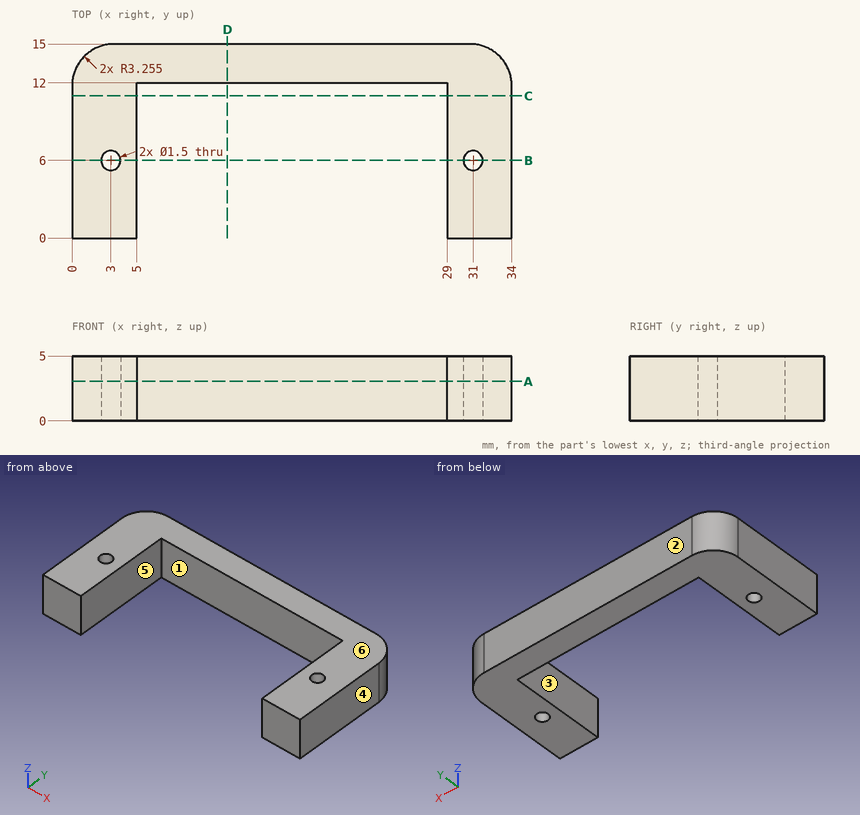
The drawing under review shows one solid part. Ordinate dimensions are in mm from its lowest x, y, z. A direction names the side the tool comes from. Give positions to 0.01 mm unless a question says otherwise; leave off trailing zeros. Order: outer loops, then holes, each group sorted by start corner. A loop starts at its lowest first (then second) coordinate and runs counter-clockwise, first axis right, second up. Notation, with made-up numbers: (66.25, -31) - (102.25, -31) arc R21 cw to (102.25, -25) - close; hole circle Ø7 at (-6.75, -29). An arc over 180 degrees is marked (long way). Answer as a JSON object with one key per item and string values. Group by question number.
Item 1: Draft analysis for pull direction X (two halves, no side actions). For the marked faces 3, 4, 5 and 6, state which applies: pulls with the +X half, pulls with the -X half, needs draft (parallel to the pull), parting line crosses it, or undercut.
Item 2: Wall thickness on line 1 along X through (y, z) = (2.75, 2.8); line 2 along Y through (x, z) = (31, 3.7); line 3 along Y through (x, z) = (7.5, 2.4): over which ranges is each line inside the solid? List them lowest first.
Item 3: Take a section at B-B on y = 6. Give the boundary of the cut face in (x, z).
Item 4: Machinability: for the marked faces 1 and 2, which of the approach directions +Z, -Z, +X, -X, +Y, -Y give a long, thin tool a straight path to every point of the face, cutting with its end or side? Answer none if there is none.
Item 5: Take a section at D-D on x = 12. Give the boundary of the cut face in (y, z).
Item 6: Clearance check with flat-ended pins moving along their axes: pin 1 Ø2 at (y, z) = (7, 4.5) entering from -X; pin 2 Ø2 at (x, z) = (18, 3.5) entering from -Y. State where each tip first meets the part, or that it passes through.
Item 7: Take a section at C-C on y = 11. Give the boundary of the cut face in (x, z), and give its area (3 significant figures).
Item 8: Take a section at A-A on z = 3.05. Give the number of separate pieces and of enclosed holes in the cut face, and give its area (3 significant figures).
Reported:
{
 "1": {"face 3": "undercut", "face 4": "pulls with the +X half", "face 5": "undercut", "face 6": "needs draft"},
 "2": {"line 1": "0 to 5, 29 to 34", "line 2": "0 to 5.25, 6.75 to 14.99", "line 3": "12 to 15"},
 "3": {"outline": "(0, 0) - (2.25, 0) - (2.25, 5) - (0, 5) - close; (3.75, 0) - (5, 0) - (5, 5) - (3.75, 5) - close; (29, 0) - (30.25, 0) - (30.25, 5) - (29, 5) - close; (31.75, 0) - (34, 0) - (34, 5) - (31.75, 5) - close"},
 "4": {"face 1": "+Z, -Z, -Y", "face 2": "+Z, -Z, +X, -X, +Y"},
 "5": {"outline": "(12, 0) - (15, 0) - (15, 5) - (12, 5) - close"},
 "6": {"pin 1": "x = 0", "pin 2": "y = 12"},
 "7": {"outline": "(0, 0) - (5, 0) - (5, 5) - (0, 5) - close; (29, 0) - (34, 0) - (34, 5) - (29, 5) - close", "area": "50.0 mm^2"},
 "8": {"separate pieces": "1", "enclosed holes": "2", "area": "214 mm^2"}
}
